Can you work these out from the model? Positions are in its coordinate system, mm. A direction names the side the tool comes from. Round coordinates to 2 decimals unless told otherwise and drop trailing zeros. Loops run counter-clockwise (first coordinate to the right, second up) from the corner with the lowest first, then second, coordinate; pieces in that order, holes last.
```python
from build123d import *

# Parameters (mm, degrees)
BOSS_START                = -91
BOSS_SKETCH_R             = 6
BOSS_DEPTH                = 6.5
INSERT_START              = -92
INSERT_HOLE_SKETCH_R      = 2.8
INSERT_HOLE_DEPTH         = 8
BOSSES_AND_HOLES_X8_COUNT = 8


with BuildPart() as part:
    # Dome Sketch → Dome (revolve)
    with BuildSketch(Plane.XY, mode=Mode.PRIVATE) as dome_sk:
        with BuildLine():
            Line((30, 97), (30, 99))
            Line((30, 99), (-0.05, 99))
            Line((-0.05, 99), (-0.05, 101.649987703))
            ThreePointArc((-0.05, 101.649987703), (-71.895079804, 71.859724464), (-101.65, 0))
            Line((-101.65, 0), (-99.65, 0))
            ThreePointArc((-99.65, 0), (-71.166784738, 69.752499955), (-2, 99.629927733))
            Line((-2, 99.629927733), (-2, 97))
            Line((-2, 97), (30, 97))
        make_face()
    revolve(dome_sk.sketch.rotate(Axis((-200, 0, 0), (1, 0, 0)), 90), axis=Axis((-200, 0, 0), (1, 0, 0)))

    # Boss Sketch → Boss (add)
    with BuildSketch(Plane(origin=(0, 0, 0), x_dir=(-1, 0, 0), z_dir=(0, -0.9238795325112867, -0.3826834323650897)).offset(BOSS_START)):
        with Locations(Location((-15, 0, 0), (0, 0, 90))):
            Circle(BOSS_SKETCH_R)
    boss = extrude(amount=-BOSS_DEPTH)

    # Insert Hole Sketch → Insert Hole (cut)
    with BuildSketch(Plane(origin=(0, 0, 0), x_dir=(-1, 0, 0), z_dir=(0, -0.9238795325112867, -0.3826834323650897)).offset(INSERT_START)):
        with Locations(Location((-15, 0, 0), (0, 0, 90))):
            Circle(INSERT_HOLE_SKETCH_R)
    insert_hole = extrude(amount=-INSERT_HOLE_DEPTH, mode=Mode.SUBTRACT)

    # Bosses and Holes x8: Boss, Insert Hole ×8 about axis
    bosses_and_holes_x8_axis = Axis((0, 0, 0), (1, 0, 0))
    add([boss.rotate(bosses_and_holes_x8_axis, i * 360 / BOSSES_AND_HOLES_X8_COUNT) for i in range(1, BOSSES_AND_HOLES_X8_COUNT)])
    add([insert_hole.rotate(bosses_and_holes_x8_axis, i * 360 / BOSSES_AND_HOLES_X8_COUNT) for i in range(1, BOSSES_AND_HOLES_X8_COUNT)], mode=Mode.SUBTRACT)


solid = part.part
```
(1) Suppose I cut it at A-A (y = 0). Write out the boundary of the cut face in (x, z), then the cut area to 3 significant figures.
(2) Which directions (+Z, -Z, +X, -X, +Y, -Y) give clear straight access to the entire face, cutting with the end or side of a thin tool? Please do faces 1 (the flat face through (15, -84, 35)), 2 (the flat face through (15, 85, -35.2)).
(3) We'd pull the mould along X, two halves only. Please class faces 3 (the flat face through (-0.05, 97, -22)), 4 (the flat face through (15, 84, 35)), 5 (the flat face through (15, 85, 35.2)): released by +X, released by -X, zero draft, split by the parting line, or undercut.
(4) For pin 1 (3 mm diameter, centred on x = -61, z = -5, fed in from -Y); pin 2 (3 mm diameter, centred on y = 45.5, z = -64.5, fed in from -X); pin 3 (12 mm diameter, centred on x = -31, z = -52.5, fed in from -Y) (3 decimals), each with a flat end and sliding along its axis, tell me the tip position at first contact or that it passes through.
(5) If I drill on line 1 (Y direction, x = 11.5, z = 0); line 2 (Z direction, x = 24.5, y = 1.5); line 3 (Z direction, x = 23, y = -85.5), over which ranges is the centre line in solid material (lowest first)?
Check result:
1. outline: (-2, -99.63) arc R99.65 cw to (-2, 99.63) - (-2, 97) - (30, 97) - (30, 99) - (-0.05, 99) - (-0.05, 101.65) arc R101.65 ccw to (-0.05, -101.65) - (-0.05, -99) - (30, -99) - (30, -97) - (-2, -97) - close
1. area: 763 mm2
2. face 1: +X
2. face 2: none
3. face 3: released by +X
3. face 4: zero draft
3. face 5: undercut
4. pin 1: stops at y = -82.27
4. pin 2: stops at x = -65.85
4. pin 3: stops at y = -85.505
5. line 1: y = -99 to -97, 97 to 99
5. line 2: z = -98.99 to -96.99, 96.99 to 98.99
5. line 3: z = -49.91 to -45.81, 45.81 to 49.91
